Autodesk Inventor part; units mm, degrees
ref_plane "YZ Plane" through (0, 0, 0) normal (1, 0, 0) x (0, 1, 0)
ref_plane "XZ Plane" through (0, 0, 0) normal (0, 1, 0) x (-1, 0, 0)
ref_plane "XY Plane" through (0, 0, 0) normal (0, 0, 1) x (1, 0, 0)
ref_plane "Work Plane1" through (0, 0, 0) normal (1, 0, 0) x (0, 1, 0)
sketch "Sketch1" plane through (0, 0, 0) normal (1, 0, 0) x (0, 1, 0)
  line L0 (0, 0) -> (5, 0) construction
  line L1 (5, 0) -> (5, 5)
  line L2 (0, 5) -> (0, 0) construction
  line L3 (0, 5) -> (5, 0)
  line L4 (0, 5) -> (5, 5)
  line L5 (5, 0) -> (0, 0) construction
  line L6 (0, 0) -> (0, 30)
  line L7 (0, 30) -> (5, 30) construction
  line L8 (5, 30) -> (5, 0)
  line L9 (0, 30) -> (5, 30)
  line L10 (5, 30) -> (5, 25)
  line L11 (5, 25) -> (0, 25)
  line L12 (0, 25) -> (0, 30)
  line L13 (0, 25) -> (5, 30)
  line L14 (0, 15) -> (5, 15) construction
  line L15 (0, 13.925) -> (5, 13.925)
  line L16 (5, 13.925) -> (5, 16.075)
  line L17 (5, 16.075) -> (0, 16.075)
  line L18 (0, 16.075) -> (0, 13.925)
  point P0 (10, 5)
  point P1 (0, 16.075)
  point P2 (0, 25)
  dimension "d4" = 5
  dimension "d10" = 30
  dimension "d11" = 5
  dimension "d12" = 5
  dimension "d13" = 5
  dimension "d14" = 5
  dimension "d15" = 1.075
  dimension "d16" = 2.15
revolve "Revolution1" add sketch "Sketch1" angle 360 about axis through (0, 0, 15) along (0, 1, 0) contours L3 L4 L1 | L4 L6 L15 L8 | L17 L6 L11 L8 | L11 L13 L8
sketch "Sketch2" plane through (0, 0, 15) normal (0, -1, 0) x (1, 0, 0)
  arc A0 (0, 1.075) -> (0, -1.075) centre (0, 0) ccw
  arc A1 (0, 10) -> (0, -10) centre (0, 0) ccw construction
  arc A2 (-9.7813, 2.08) -> (-9.7813, -2.08) centre (0, 0) ccw
  arc A3 (-15.2728, 0.745) -> (-15.2761, -0.675) centre (0, 0) ccw
  arc A4 (-15.2761, -0.675) -> (-9.7813, -2.08) centre (-9.8343, 9.1599) ccw
  arc A5 (-9.7813, 2.08) -> (-15.2728, 0.745) centre (-9.9572, -9.1586) ccw
  point P0 (0, -15)
  dimension "d17" = 4.16
  dimension "d18" = 2.08
  dimension "d21" = 0.745
  dimension "d22" = 1.42
  dimension "d23" = 15.291
  dimension "d24" = 11.24
  dimension "d25" = 11.24
sketch "Sketch3" plane through (0, 5, 15) normal (0, 1, 0) x (1, 0, 0)
  arc A0 (0, 1.075) -> (0, -1.075) centre (0, 0) ccw
  arc A1 (0, 15) -> (0, -15) centre (0, 0) ccw
  arc A2 (-14.714, 2.915) -> (-14.714, -2.915) centre (0, 0) ccw
  arc A3 (-21.0975, 0.975) -> (-21.0975, -0.975) centre (0, 0) ccw
  arc A4 (-21.0975, -0.975) -> (-14.714, -2.915) centre (-14.5146, 9.2134) ccw
  arc A5 (-14.714, 2.915) -> (-21.0975, 0.975) centre (-14.5146, -9.2134) ccw
  dimension "d26" = 2.915
  dimension "d27" = 5.83
  dimension "d29" = 0.975
  dimension "d30" = 1.95
  dimension "d31" = 15
  dimension "d32" = 21.12
  dimension "d33" = 12.13
  dimension "d34" = 12.13
loft "Loft1" add profiles "Sketch2", "Sketch3"
pattern_circular "Circular Pattern1" count 10 over 360 about axis through (0, 2.5, 15) along (0, 1, 0) of "Loft1"
equation "\"t\" = 0.15"
properties part number "bevelGear"
Geometry: final body of the model. Coordinates: model frame, mm. A direction names the side the tool comes from. Coordinates: 2 decimals unless noted, no trailing zeros. Loops run counter-clockwise (first coordinate to the right, second up) from the corner with the lowest first, then second, coordinate; pieces in that order, holes last. Notation, with made-up numbers: M 61,84.25 L 84,84.25 A31 ccw 84,118.25 Z; hole C 53,23 d4. An arc over 180 degrees is marked long. Put each result on its own line as item: value.
(1) Cut plane A-A on x = 0. Return the cut outline in (y, z) (3 decimals), then the cut area to 3 significant figures.
Answer sheet:
outline: M 0,5 L 5,0 L 5,13.925 L 0,13.925 Z; M 0,16.075 L 5,16.075 L 5,30 L 0,25 Z
area: 114 mm^2
(2) First-contact query: pin 1 (1.5 mm diameter, centred on x = -5.5, y = 3, fed in from -Z); pin 2 (1.5 mm diameter, centred on y = 4, z = 22, fed in from -X). Flat tips, straight axial feed; report the tip coordinate or a pass-through.
Answer sheet:
pin 1: stops at z = -3.9
pin 2: stops at x = -14.84
(3) Material intervals for probe 1 along Z at (x, y) = (-11.5, 1.5); probe 2 along X at (y, z) = (1.3, 6); probe 3 along Z at (x, y) = (13.5, 1.1), sorted ascending.
Answer sheet:
probe 1: z = 4.71 to 9.44, 12.67 to 17.33, 20.57 to 25.32
probe 2: x = -13.95 to -8.58, -6.83 to 6.83, 8.57 to 13.91
probe 3: z = 5.39 to 6.55, 13.02 to 16.95, 23.37 to 24.61
(4) Access query for faces 5 (the face through (-7.351, 2.535, 4.847)), 6 (the face through (11.92, 2.54, 18.89)), 7 (the face through (-11.92, 2.54, 11.11)). Directions: +Z, -Z, +X, -X, +Y, -Y. A direction counts if a zero-diameter tool reaches every point of the face in a straight line with its end or side. Return the directions, or none.
Answer sheet:
face 5: -Y
face 6: +X, -Y
face 7: -X, -Y
(5) Draft query along X for faces 1 (the face through (7.351, 2.535, 25.153)), 2 (the face through (-11.928, 2.535, 18.854)), 3 (the face through (11.928, 2.535, 11.146)), 4 (the face through (-7.385, 2.535, 25.129)). Return one class per face: pulls with the +X half, pulls with the -X half, needs draft (parallel to the pull), parting line crosses it, or undercut.
Answer sheet:
face 1: undercut
face 2: pulls with the -X half
face 3: pulls with the +X half
face 4: undercut
